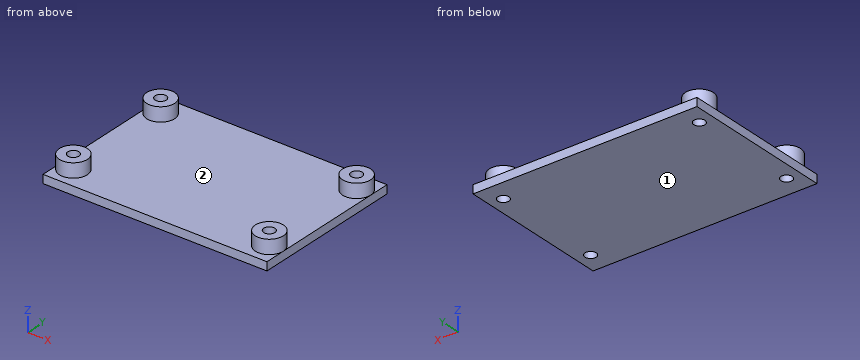
```python
from build123d import *

# Parameters (mm, degrees)
SKETCH_W     = 80
SKETCH_H     = 55
PAD_DEPTH    = 3
SKETCH001_R  = 5
PAD001_DEPTH = 5
SKETCH002_R  = 2
POCKET_DEPTH = 5


with BuildPart() as part:
    # Sketch → Pad (new body)
    with BuildSketch(Plane.XY):
        with Locations((40, 27.5)):
            Rectangle(SKETCH_W, SKETCH_H)
    extrude(amount=-PAD_DEPTH)

    # Sketch001 → Pad001 (join)
    with BuildSketch(Plane.XY):
        with Locations((5, 47.5)):
            Circle(SKETCH001_R)
        with Locations((75, 47.5)):
            Circle(SKETCH001_R)
        with Locations((5, 7.5)):
            Circle(SKETCH001_R)
        with Locations((75, 7.5)):
            Circle(SKETCH001_R)
    extrude(amount=PAD001_DEPTH)

    # Sketch002 → Pocket (cut, symmetric)
    with BuildSketch(Plane.XY):
        with Locations((5, 47.5)):
            Circle(SKETCH002_R)
        with Locations((75, 47.5)):
            Circle(SKETCH002_R)
        with Locations((75, 7.5)):
            Circle(SKETCH002_R)
        with Locations((5, 7.5)):
            Circle(SKETCH002_R)
    extrude(amount=POCKET_DEPTH, both=True, mode=Mode.SUBTRACT)


solid = part.part
```
Input: part model. Units: mm. Frame: model coordinates. Face numbers are marked on the shaded views. Coordinates: 2 decimals unless noted, no trailing zeros. Order: outer loops, then holes, each group sorted by start corner. A loop starts at its lowest first (then second) coordinate and runs counter-clockwise, first axis right, second up. Notation, with made-up numbers: (13, 59.5) - (72, 59.5) arc R7 ccw to (72, 68.5) - close; hole circle Ø4 at (30, 63.25). An arc over 180 degrees is marked (long way). Put each result on its own line as item: value.
1. Line query: line 1 along Y through (x, z) = (5, -2.35); line 2 along Y through (x, z) = (75, 1.2); line 3 along Y through (x, z) = (74.5, -1.25). Output: solid intervals per line, ascending.
Report:
line 1: y = 0 to 5.5, 9.5 to 45.5, 49.5 to 55
line 2: y = 2.5 to 5.5, 9.5 to 12.5, 42.5 to 45.5, 49.5 to 52.5
line 3: y = 0 to 5.56, 9.44 to 45.56, 49.44 to 55
2. Cut plane A-A on x = 75. Return the cut outline in (y, z).
Report:
outline: (0, -3) - (5.5, -3) - (5.5, 5) - (2.5, 5) - (2.5, 0) - (0, 0) - close; (9.5, -3) - (45.5, -3) - (45.5, 5) - (42.5, 5) - (42.5, 0) - (12.5, 0) - (12.5, 5) - (9.5, 5) - close; (49.5, -3) - (55, -3) - (55, 0) - (52.5, 0) - (52.5, 5) - (49.5, 5) - close
3. Cut plane C-C on x = 31. Return the cut outline in (y, z).
Report:
outline: (0, -3) - (55, -3) - (55, 0) - (0, 0) - close
4. Cut plane B-B on y = 27. Return the cut outline in (x, z), then the cut area to 3 significant figures.
Report:
outline: (0, -3) - (80, -3) - (80, 0) - (0, 0) - close
area: 240 mm2
5. Draft query along Y for the marked faces 1 and 2. Return one class per face: pulls with the +Y half, pulls with the -Y half, needs draft (parallel to the pull), parting line crosses it, or undercut.
Report:
face 1: needs draft
face 2: undercut
6. Contact query for flat-ended pins moving along their axis: pin 1 Ø5 at (x, y) = (5, 47.5) entering from +Z; pin 2 Ø3 at (x, y) = (75, 47.5) entering from -Z; pin 3 Ø2 at (x, y) = (16, 23.5) entering from +Z. Output: stop coordinate, or through.
Report:
pin 1: stops at z = 5
pin 2: passes through
pin 3: stops at z = 0
